Geometry: final body of the model. Coordinates: model frame, mm. Face numbers are marked on the shaded views. A direction names the side the tool comes from. Round coordinates to 2 decimals unless told otherwise and drop trailing zeros. Order: outer loops, then holes, each group sorted by start corner. A loop starts at its lowest first (then second) coordinate and runs counter-clockwise, first axis right, second up. Notation, with made-up numbers: M -13,38.5 L 34,38.5 A31 ccw 34,71.5 Z; hole C 84.5,53 d9. An arc over 180 degrees is marked long. Return JSON: item names as keys, results as strings. Group by question number.
Q1. Ray query, probe 1 along X at (y, z) = (3.25, 0); probe 2 along X at (y, z) = (5.75, 0); probe 3 along Y at (x, z) = (49, -9). Return the intervals inside material, ascending.
Q2. Mould query, pull axis X, two halves, no side actions, for the marked faces 3 and 4. Classes: released by +X, released by -X, zero draft, split by the parting line, or undercut.
Q3. Cut plane D-D on x = 11. Output: boundary loops of the cut face in (y, z), and give its area (3 significant figures).
Q4. Contact query for flat-ended pins moving along their axis: pin 1 (1 mm diameter, centred on x = 42, z = -5.5, fed in from +Y); pin 2 (5 mm diameter, centred on y = 4.5, z = -9.5, fed in from +X); pin 3 (1.5 mm diameter, centred on y = 5, z = 6.5, fed in from +X). Output: stop coordinate, or through.
Q5. Cut plane A-A on z = 0. Output: boundary loops of the cut face in (x, y), and give its area (3 significant figures).
Q6. Access query for the marked faces 1 and 2. Directions: +Z, -Z, +X, -X, +Y, -Y. A direction counts if a zero-diameter tool reaches every point of the face in a straight line with its end or side. Return the directions, or none.
Q7. Cut plane C-C on z = -10. Output: boundary loops of the cut face in (x, y).
Q8. Cut plane B-B on y = 3.25. Output: boundary loops of the cut face in (x, z).
```python
from build123d import *
from build123d.topology import SkipClean

# Parameters (mm, degrees)
EXTRUDE_1_DEPTH     = 5
SKETCH_5_R          = 12.5
EXTRUDE_2_DEPTH     = 2
CUT_EXTRUDE_1_REACH = 80.813
SKETCH_6_R          = 2.5
SKETCH_8_R          = 12.5
EXTRUDE_3_DEPTH     = 4.6
CUT_EXTRUDE_2_REACH = 81.086
SKETCH_7_R          = 2.5


with BuildPart() as part:
    # Sketch 1 → Extrude 1 (new body)
    with BuildSketch(Plane(origin=(0, 0, 0), x_dir=(1, 0, 0), z_dir=(0, 1, 0))):
        with BuildLine():
            Line((-65, 12.5), (65, 12.5))
            ThreePointArc((65, 12.5), (77.5, 0), (65, -12.5))
            Line((65, -12.5), (-65, -12.5))
            ThreePointArc((-65, -12.5), (-77.5, 0), (-65, 12.5))
        make_face()
    extrude(amount=EXTRUDE_1_DEPTH)

    # Sketch 5 → Extrude 2 (add)
    with SkipClean():  # the faces are left unmerged after this step: merging them gives an invalid solid
        with BuildSketch(Plane(origin=(0, 5, 0), x_dir=(1, 0, 0), z_dir=(0, 1, 0))):
            with Locations(Location((-65, 0, 0), (0, 0, 270))):
                Circle(SKETCH_5_R)
        extrude(amount=EXTRUDE_2_DEPTH)

    # Sketch 6 → Cut-Extrude 1 (cut, up to next)
    with BuildSketch(Plane(origin=(0, 7, 0), x_dir=(1, 0, 0), z_dir=(0, 1, 0)), mode=Mode.PRIVATE) as cut_extrude_1_sk1:
        with Locations(Location((-65, 0, 0), (0, 0, 270))):
            Circle(SKETCH_6_R)
    cut_extrude_1_tool1 = extrude(cut_extrude_1_sk1.sketch, amount=-CUT_EXTRUDE_1_REACH, mode=Mode.PRIVATE) & part.part
    add(cut_extrude_1_tool1.solids().sort_by_distance((-65, 7, 0))[0], mode=Mode.SUBTRACT)

    # Sketch 8 → Extrude 3 (add)
    with SkipClean():  # the faces are left unmerged after this step: merging them gives an invalid solid
        with BuildSketch(Plane(origin=(0, 5, 0), x_dir=(1, 0, 0), z_dir=(0, 1, 0))):
            with Locations(Location((65, 0, 0), (0, 0, 270))):
                Circle(SKETCH_8_R)
        extrude(amount=EXTRUDE_3_DEPTH)
    add(part.part.scale(1), mode=Mode.REPLACE)  # the faces are merged on a copy

    # Sketch 7 → Cut-Extrude 2 (cut, up to next)
    with BuildSketch(Plane(origin=(0, 9.6, 0), x_dir=(1, 0, 0), z_dir=(0, 1, 0)), mode=Mode.PRIVATE) as cut_extrude_2_sk1:
        with Locations(Location((65, 0, 0), (0, 0, 270))):
            Circle(SKETCH_7_R)
    cut_extrude_2_tool1 = extrude(cut_extrude_2_sk1.sketch, amount=-CUT_EXTRUDE_2_REACH, mode=Mode.PRIVATE) & part.part
    add(cut_extrude_2_tool1.solids().sort_by_distance((65, 9.6, 0))[0], mode=Mode.SUBTRACT)


solid = part.part
```
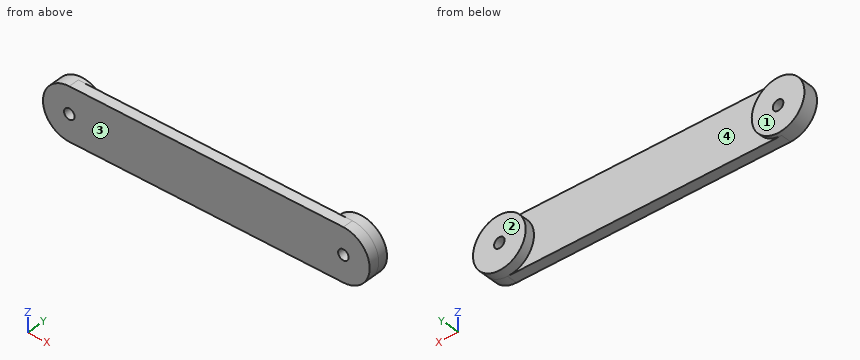
Result sheet:
{
 "1": {"probe 1": "x = -77.5 to -67.5, -62.5 to 62.5, 67.5 to 77.5", "probe 2": "x = -77.5 to -67.5, -62.5 to -52.5, 52.5 to 62.5, 67.5 to 77.5", "probe 3": "y = 0 to 5"},
 "2": {"face 3": "zero draft", "face 4": "undercut"},
 "3": {"outline": "M 0,-12.5 L 5,-12.5 L 5,12.5 L 0,12.5 Z", "area": "125 mm²"},
 "4": {"pin 1": "stops at y = 5", "pin 2": "stops at x = 75.36", "pin 3": "stops at x = 76.1"},
 "5": {"outline": "M -77.5,0 L -67.5,0 L -67.5,7 L -77.5,7 Z; M -62.5,0 L 62.5,0 L 62.5,9.6 L 52.5,9.6 L 52.5,5 L -52.5,5 L -52.5,7 L -62.5,7 Z; M 67.5,0 L 77.5,0 L 77.5,9.6 L 67.5,9.6 Z", "area": "857 mm²"},
 "6": {"face 1": "+Z, -Z, -X, +Y", "face 2": "+Z, -Z, +X, -X, +Y"},
 "7": {"outline": "M -72.5,0 L 72.5,0 L 72.5,9.6 L 57.5,9.6 L 57.5,5 L -57.5,5 L -57.5,7 L -72.5,7 Z"},
 "8": {"outline": "M -65,-12.5 L 65,-12.5 A12.5 ccw 65,12.5 L -65,12.5 A12.5 ccw Z; hole C -65,0 d5; hole C 65,0 d5"}
}
